```python
from build123d import *

# Parameters (mm, degrees)
SKETCH1_R           = 10
BOSS_EXTRUDE1_DEPTH = 4
SKETCH2_R           = 3
BOSS_EXTRUDE2_DEPTH = 80
CUT_EXTRUDE1_DEPTH  = 2


with BuildPart() as part:
    # Sketch1 → Boss-Extrude1 (new body)
    with BuildSketch(Plane.XY):
        Circle(SKETCH1_R)
    extrude(amount=BOSS_EXTRUDE1_DEPTH)

    # Sketch2 → Boss-Extrude2 (add)
    with BuildSketch(Plane.XY.offset(4)):
        Circle(SKETCH2_R)
    extrude(amount=BOSS_EXTRUDE2_DEPTH)

    # Sketch3 → Cut-Extrude1 (cut)
    with BuildSketch(Plane(origin=(0, 0, 0), x_dir=(-1, 0, 0), z_dir=(0, 0, -1))):
        Polygon((-4.148384256, 7.097061567), (-8.220427737, -0.044075367), (-4.072043481, -7.141136934), (4.148384256, -7.097061567), (8.220427737, 0.044075367), (4.072043481, 7.141136934), align=None)
    extrude(amount=-CUT_EXTRUDE1_DEPTH, mode=Mode.SUBTRACT)


solid = part.part
```
Could you check a few things on this model? Use its own coordinates, in mm. A direction names the side the tool comes from. Round coordinates to 2 decimals unless told otherwise and drop trailing zeros. Write each loop counter-clockwise with the first axis right and the second up, starting at its lowest first coordinate (ties: lowest second). Pieces come first, ordered by that corner, then holes.
(1) For pin 1 (4.5 mm diameter, centred on x = 2.5, y = 0, fed in from -Z); pin 2 (10 mm diameter, centred on x = 4.5, y = -7.5, fed in from +Z); pin 3 (10 mm diameter, centred on x = 5, y = -1.5, fed in from -Z); pin 4 (6 mm diameter, centred on x = -8, z = 36.5, fed in from -Y), each with a flat end and sliding along its axis, tell me the tip position at first contact or that it passes through.
Findings below:
pin 1: stops at z = 2
pin 2: stops at z = 4
pin 3: stops at z = 0
pin 4: passes through
(2) If I drill on probe 1 along Z at (x, y) = (0.75, -1.75); probe 2 along Z at (x, y) = (-5.5, -8); probe 3 along Y at (x, z) = (0.75, 70.5), over which ranges is the centre line in solid material (lowest first)?
Findings below:
probe 1: z = 2 to 84
probe 2: z = 0 to 4
probe 3: y = -2.9 to 2.9
(3) Suppose I cut it at C-C on z = 22.5. Write out the boundary of the cut face in (x, y), and give its area (3 significant figures).
Findings below:
outline: circle Ø6 at (0, 0)
area: 28.3 mm2
(4) Thinking about a two-plate mould opening in X: for faces 1 (the face through (-2.17, -9.76, 1.97)), 2 (the face through (2.1, 2.4, 4)), 3 (the face through (6.156, 3.576, 0.986)), 4 (the face through (-6.2, 3.5, 1)), which applies, +X half, -X half, draft (parallel to the pull), parting line (faces both ways), or undercut?
Findings below:
face 1: parting line
face 2: draft
face 3: undercut
face 4: undercut
(5) Suppose I cut it at B-B on x = -2. Write out the boundary of the cut face in (y, z).
Findings below:
outline: (-9.8, 0) - (-7.11, 0) - (-7.11, 2) - (7.13, 2) - (7.13, 0) - (9.8, 0) - (9.8, 4) - (2.24, 4) - (2.24, 84) - (-2.24, 84) - (-2.24, 4) - (-9.8, 4) - close
(6) Suppose I cut it at A-A on y = -6.25. Write out the boundary of the cut face in (x, z).
Findings below:
outline: (-7.81, 0) - (-4.63, 0) - (-4.63, 2) - (4.59, 2) - (4.59, 0) - (7.81, 0) - (7.81, 4) - (-7.81, 4) - close
(7) Suppose I cut it at D-D on x = 7.5. Write out the boundary of the cut face in (y, z), and give its area (3 significant figures).
Findings below:
outline: (-6.61, 0) - (-1.28, 0) - (-1.28, 2) - (1.22, 2) - (1.22, 0) - (6.61, 0) - (6.61, 4) - (-6.61, 4) - close
area: 47.9 mm2
(8) Which directions (+Z, -Z, +X, -X, +Y, -Y) give clear straight access to the entire face, cutting with the end or side of a thin tool? Please do faces 5 (the face through (-3, 0, 43)), 6 (the face through (0, 0, 2)), 7 (the face through (7, 3, 0)).
Findings below:
face 5: +Z
face 6: -Z
face 7: -Z, +X, -X, +Y, -Y
